Verification items for the finished model (mm, model axes). A direction names the side the tool comes from. Give positions to 0.01 mm unless a question says otherwise; leave off trailing zeros. Order: outer loops, then holes, each group sorted by start corner. A loop starts at its lowest first (then second) coordinate and runs counter-clockwise, first axis right, second up. Notation, with made-up numbers: (19.25, 36.5) - (41.25, 36.5) arc R16 cw to (41.25, 61.5) - close; hole circle Ø3 at (89.25, 17.25). An arc over 180 degrees is marked (long way). Answer as a JSON object with one key per item and string values.
```python
from build123d import *

# Parameters (mm, degrees)
SKETCH1_R           = 0.8
BOSS_EXTRUDE1_DEPTH = 3
FILLET1_R           = 6
SKETCH2_R           = 2
CUT_EXTRUDE1_DEPTH  = 3
BOSS_EXTRUDE2_START = 1.5
SKETCH3_R           = 4
SKETCH3_R_2         = 2
BOSS_EXTRUDE2_DEPTH = 1.5
SKETCH4_R           = 1
CUT_EXTRUDE2_DEPTH  = 3


with BuildPart() as part:
    # Sketch1 → Boss-Extrude1 (new body)
    # profile 1 of 2: a face of its own
    with BuildSketch(Plane.XY):
        with BuildLine():
            Line((25, -3), (-25, -3))
            ThreePointArc((-25, -3), (-28, 0), (-25, 3))
            Line((-25, 3), (25, 3))
            ThreePointArc((25, 3), (28, 0), (25, -3))
        make_face()
        with Locations((-6, 0)):
            Circle(SKETCH1_R, mode=Mode.SUBTRACT)
        with Locations((6, 0)):
            Circle(SKETCH1_R, mode=Mode.SUBTRACT)
    # profile 2 of 2: a face of its own
    with BuildSketch(Plane.XY):
        with BuildLine():
            Line((-3, -25), (-3, 25))
            ThreePointArc((-3, 25), (0, 28), (3, 25))
            Line((3, 25), (3, -25))
            ThreePointArc((3, -25), (0, -28), (-3, -25))
        make_face()
        with Locations((0, 6)):
            Circle(SKETCH1_R, mode=Mode.SUBTRACT)
        with Locations((0, -6)):
            Circle(SKETCH1_R, mode=Mode.SUBTRACT)
    extrude(amount=BOSS_EXTRUDE1_DEPTH)

    # Fillet1
    fillet1_edges = [part.edges().sort_by_distance(p)[0] for p in [
        (3, -3, 1.5),
        (-3, -3, 1.5),
        (-3, 3, 1.5),
        (3, 3, 1.5),
    ]]
    fillet(fillet1_edges, radius=FILLET1_R)

    # Sketch2 → Cut-Extrude1 (cut)
    with BuildSketch(Plane.XY.offset(3)):
        Circle(SKETCH2_R)
    extrude(amount=-CUT_EXTRUDE1_DEPTH, mode=Mode.SUBTRACT)

    # Sketch3 → Boss-Extrude2 (add)
    with BuildSketch(Plane.XY.offset(3).offset(BOSS_EXTRUDE2_START)):
        Circle(SKETCH3_R)
        Circle(SKETCH3_R_2, mode=Mode.SUBTRACT)
    extrude(amount=-BOSS_EXTRUDE2_DEPTH)

    # Sketch4 → Cut-Extrude2 (cut)
    with BuildSketch(Plane.XY.offset(3)):
        with Locations((0, 25)):
            Circle(SKETCH4_R)
        with Locations((25, 0)):
            Circle(SKETCH4_R)
        with Locations((0, -25)):
            Circle(SKETCH4_R)
        with Locations((-25, 0)):
            Circle(SKETCH4_R)
    extrude(amount=-CUT_EXTRUDE2_DEPTH, mode=Mode.SUBTRACT)


solid = part.part
```
(1) Release check for a two-part mould opening along Y. For faces 1 (the cylindrical face through (-0.104, 6.793, 1.479)), 2 (the flat face through (-3, -17, 1)), 3 (the flat face through (-17, 3, 1)), 4 (the cylindrical face through (-26, 0, 2)) record: pulls with the +Y half, pulls with the -Y half, needs draft (parallel to the pull), parting line crosses it, or undercut.
Computed values:
{"face 1": "undercut", "face 2": "needs draft", "face 3": "pulls with the +Y half", "face 4": "undercut"}
(2) Gauge pin test, flat ends, axial feed: pin 1 Ø2.5 at (x, z) = (19.5, 1) entering from +Y; pin 2 Ø1.5 at (x, z) = (-21, 1) entering from -Y; pin 3 Ø2.5 at (x, y) = (0, -25) entering from +Z; pin 4 Ø1.8 at (x, y) = (0, -6) entering from -Z. Record the tip position at first contact, or that the pin passes through.
Computed values:
{"pin 1": "stops at y = 3", "pin 2": "stops at y = -3", "pin 3": "stops at z = 3", "pin 4": "stops at z = 0"}
(3) Material ranges on line 1 along Y through (x, z) = (0, 1.85); line 2 along Y through (x, z) = (-25, 2.35); line 3 along X through (y, z) = (17.5, 1.05), recorded low to high. Write a range as [from, to].
Computed values:
{"line 1": "y = [-28, -26], [-24, -6.8], [-5.2, -2], [2, 5.2], [6.8, 24], [26, 28]", "line 2": "y = [-3, -1], [1, 3]", "line 3": "x = [-3, 3]"}
(4) Access from +Z, -Z, +X, -X, +Y, -Y to the whole of each face (thin tool, end or side, straight path). Record for faces 5 (the flat face through (4.3, 0.1, 3)), 6 (the flat face through (17, 3, 1)), 7 (the flat face through (-17, -3, 1)), 8 (the flat face through (-3, 17, 1)), 9 (the flat face through (17, -3, 1)).
Computed values:
{"face 5": "+Z", "face 6": "+Z, -Z, +X, +Y", "face 7": "+Z, -Z, -X, -Y", "face 8": "+Z, -Z, -X, +Y", "face 9": "+Z, -Z, +X, -Y"}
(5) Section check C-C (z = 1.65). Count the separate pieces of the cut face and the enclosed holes in it, then the cut area to 3 significant figures.
Computed values:
{"separate pieces": "1", "enclosed holes": "9", "area": "618 mm²"}
(6) Section check A-A (x = 0). Record the cut outline in (y, z).
Computed values:
{"outline": "(-28, 0) - (-26, 0) - (-26, 3) - (-28, 3) - close; (-24, 0) - (-6.8, 0) - (-6.8, 3) - (-24, 3) - close; (-5.2, 0) - (-2, 0) - (-2, 4.5) - (-4, 4.5) - (-4, 3) - (-5.2, 3) - close; (2, 0) - (5.2, 0) - (5.2, 3) - (4, 3) - (4, 4.5) - (2, 4.5) - close; (6.8, 0) - (24, 0) - (24, 3) - (6.8, 3) - close; (26, 0) - (28, 0) - (28, 3) - (26, 3) - close"}
(7) Section check D-D (y = 6). Record the cut outline in (x, z), then the cut area to 3 significant figures.
Computed values:
{"outline": "(-3.8, 0) - (-0.8, 0) - (-0.8, 3) - (-3.8, 3) - close; (0.8, 0) - (3.8, 0) - (3.8, 3) - (0.8, 3) - close", "area": "18.0 mm²"}
